Geometry check sheet. Reference: the model listing, model coordinates, mm. Give positions to 0.01 mm unless a question says otherwise; leave off trailing zeros. Loops run counter-clockwise (first coordinate to the right, second up) from the corner with the lowest first, then second, coordinate; pieces in that order, holes last. Notation, with made-up numbers: (-24.75, 23) - (16.25, 23) arc R23 ccw to (16.25, 39) - close; hole circle Ø10 at (-25.75, 32). An arc over 180 degrees is marked (long way). Use a Markdown table: item, result. Add a question column.
1. Cross-section at A-A on x = 7. Enter the section's corners in (y, z).
2. Cross-section at C-C on y = -0.25. Enter the section's corners in (x, z).
3. Depth check by flat-ended pin: P1, Ø2, axis at y = -1, z = 0, coming from the -X side; P2, Ø2, axis at x = 5, y = -2.5, coming from the -Z side. Enter the tip coordinate at first touch or a pass-through.
4. Material ranges on L1, parallel to Z at x = 0, y = 2; L2, parallel to Y at x = -1.25, z = -0.75 (3 decimals), recorded low to high.
5. Cross-section at B-B on z = -1.25. Count the separate pieces of the cut face and the enclosed holes in it, and give its area (3 significant figures).
6. Cross-section at D-D on x = 0. Enter the section's corners in (y, z), and give its area (3 significant figures).
7. Draft check along Y on faces 1 (the flat face through (10.1, 0, 6)), 2 (the flat face through (0, 0, 0.5)), 3 (the flat face through (0, 5, 6)). Enter one of: pulls with the +Y half, pulls with the -Y half, needs draft (parallel to the pull), parting line crosses it, or undercut.
from build123d import *

# Parameters (mm, degrees)
SKETCH1_W            = 20.2
SKETCH1_H            = 10
BOSS_EXTRUDE1_DEPTH  = 11.5
SKETCH2_W            = 13
SKETCH2_H            = 10
SKETCH2_W_2          = 1.525
CUT_EXTRUDE1_DEPTH   = 0.5
SKETCH3_W            = 17.15
SKETCH3_H            = 9.56
CUT_EXTRUDE2_DEPTH   = 0.5
SKETCH4_W            = 0.48
SKETCH4_H            = 0.27
BOSS_EXTRUDE2_DEPTH  = 3.5
FILLET1_R            = 0.06
FILLET1_OF_MIRROR1_R = 0.06
FILLET2_R            = 0.05


with BuildPart() as part:
    # Sketch1 → Boss-Extrude1 (new body)
    with BuildSketch(Plane.XY):
        Rectangle(SKETCH1_W, SKETCH1_H)
    extrude(amount=BOSS_EXTRUDE1_DEPTH)

    # Sketch2 → Cut-Extrude1 (cut)
    with BuildSketch(Plane(origin=(0, 0, 0), x_dir=(-1, 0, 0), z_dir=(0, 0, -1))):
        Rectangle(SKETCH2_W, SKETCH2_H)
        with Locations((-9.3375, 0)):
            Rectangle(SKETCH2_W_2, SKETCH2_H)
        with Locations((9.3375, 0)):
            Rectangle(SKETCH2_W_2, SKETCH2_H)
    extrude(amount=-CUT_EXTRUDE1_DEPTH, mode=Mode.SUBTRACT)

    # Sketch3 → Cut-Extrude2 (cut)
    with BuildSketch(Plane(origin=(0, 0, 0), x_dir=(-1, 0, 0), z_dir=(0, 0, -1))):
        Rectangle(SKETCH3_W, SKETCH3_H)
    extrude(amount=-CUT_EXTRUDE2_DEPTH, mode=Mode.SUBTRACT)

    # Sketch4 → Boss-Extrude2 (add)
    with BuildSketch(Plane(origin=(0, 0, 0.5), x_dir=(-1, 0, 0), z_dir=(0, 0, -1))):
        with Locations((8.9, -3.81)):
            Rectangle(SKETCH4_W, SKETCH4_H)
        with Locations((1.28, -3.81)):
            Rectangle(SKETCH4_W, SKETCH4_H)
        with Locations((-3.8, -3.81)):
            Rectangle(SKETCH4_W, SKETCH4_H)
        with Locations((-8.88, -3.81)):
            Rectangle(SKETCH4_W, SKETCH4_H)
    boss_extrude2 = extrude(amount=BOSS_EXTRUDE2_DEPTH)

    # Fillet1
    fillet1_edges = [part.edges().sort_by_distance(p)[0] for p in [
        (-1.52, -3.675, -1.25),
        (-1.52, -3.945, -1.25),
        (-1.04, -3.945, -1.25),
        (-1.04, -3.675, -1.25),
        (3.56, -3.675, -1.25),
        (3.56, -3.945, -1.25),
        (4.04, -3.945, -1.25),
        (4.04, -3.675, -1.25),
        (8.64, -3.675, -1.25),
        (8.64, -3.945, -1.25),
        (9.12, -3.945, -1.25),
        (9.12, -3.675, -1.25),
        (-9.14, -3.675, -1.25),
        (-9.14, -3.945, -1.25),
        (-8.66, -3.945, -1.25),
        (-8.66, -3.675, -1.25),
    ]]
    fillet(fillet1_edges, radius=FILLET1_R)

    # Mirror1: Boss-Extrude2 across plane
    add(boss_extrude2.mirror(Plane.ZX))

    # Fillet1 of Mirror1
    fillet1_of_mirror1_edges = [part.edges().sort_by_distance(p)[0] for p in [
        (-1.52, 3.675, -1.25),
        (-1.52, 3.945, -1.25),
        (-1.04, 3.945, -1.25),
        (-1.04, 3.675, -1.25),
        (3.56, 3.675, -1.25),
        (3.56, 3.945, -1.25),
        (4.04, 3.945, -1.25),
        (4.04, 3.675, -1.25),
        (8.64, 3.675, -1.25),
        (8.64, 3.945, -1.25),
        (9.12, 3.945, -1.25),
        (9.12, 3.675, -1.25),
        (-9.14, 3.675, -1.25),
        (-9.14, 3.945, -1.25),
        (-8.66, 3.945, -1.25),
        (-8.66, 3.675, -1.25),
    ]]
    fillet(fillet1_of_mirror1_edges, radius=FILLET1_OF_MIRROR1_R)

    # Fillet2
    fillet2_edges = [part.edges().sort_by_distance(p)[0] for p in [
        (-10.1, 0, 11.5),
        (0, -5, 11.5),
        (10.1, 0, 11.5),
        (0, 5, 11.5),
        (10.1, -5, 6),
        (-10.1, -5, 6),
        (-10.1, 5, 6),
        (10.1, 5, 6),
    ]]
    fillet(fillet2_edges, radius=FILLET2_R)


solid = part.part
Values found:
| question | item | result |
|---|---|---|
| 1 | outline | (-5, 0) - (-4.78, 0) - (-4.78, 0.5) - (4.78, 0.5) - (4.78, 0) - (5, 0) - (5, 11.45) arc R0.05 ccw to (4.95, 11.5) - (-4.95, 11.5) arc R0.05 ccw to (-5, 11.45) - close |
| 2 | outline | (-10.1, 0.5) - (10.1, 0.5) - (10.1, 11.45) arc R0.05 ccw to (10.05, 11.5) - (-10.05, 11.5) arc R0.05 ccw to (-10.1, 11.45) - close |
| 3 | P1 | stops at x = -10.1 |
| 3 | P2 | stops at z = 0.5 |
| 4 | L1 | z = 0.5 to 11.5 |
| 4 | L2 | y = -3.945 to -3.675, 3.675 to 3.945 |
| 5 | separate pieces | 8 |
| 5 | enclosed holes | 0 |
| 5 | area | 1.01 mm2 |
| 6 | outline | (-5, 0.5) - (5, 0.5) - (5, 11.45) arc R0.05 ccw to (4.95, 11.5) - (-4.95, 11.5) arc R0.05 ccw to (-5, 11.45) - close |
| 6 | area | 110 mm2 |
| 7 | face 1 | needs draft |
| 7 | face 2 | undercut |
| 7 | face 3 | pulls with the +Y half |
